from build123d import *

# Parameters (mm, degrees)
SKETCH1_W            = 15.8
SKETCH1_H            = 3.2
BOSS_EXTRUDE1_DEPTH  = 7.8
SKETCH2_R            = 2.4
BOSS_EXTRUDE2_DEPTH  = 1.6
LPATTERN1_COUNT      = 2
LPATTERN1_PITCH      = 8
LPATTERN1_COUNT_DIR2 = 6
LPATTERN1_PITCH_DIR2 = 8
SHELL1_T             = -1.2
SKETCH3_R            = 1.5
SKETCH3_R_2          = 0.6
BOSS_EXTRUDE3_DEPTH  = 1.8
BOSS_EXTRUDE4_DEPTH  = 1.5
SKETCH5_R            = 2.4
SKETCH5_R_2          = 1.55
BOSS_EXTRUDE5_DEPTH  = 1.6
LPATTERN2_COUNT      = 4
LPATTERN2_PITCH      = 8


with BuildPart() as part:
    # Sketch1 → Boss-Extrude1 (new body)
    with BuildSketch(Plane.XY):
        with Locations((7.9, 1.6)):
            Rectangle(SKETCH1_W, SKETCH1_H)
    extrude(amount=-BOSS_EXTRUDE1_DEPTH)

    # Sketch2 → Boss-Extrude2 (add)
    with BuildSketch(Plane(origin=(0, 3.2, 0), x_dir=(1, 0, 0), z_dir=(0, 1, 0))):
        with Locations(Location((3.9, 3.9, 0), (0, 0, 270))):
            Circle(SKETCH2_R)
    boss_extrude2 = extrude(amount=BOSS_EXTRUDE2_DEPTH)

    # LPattern1: Boss-Extrude2 2 × 6, 10 skipped
    with Locations(*[(j * LPATTERN1_PITCH_DIR2, 0, i * LPATTERN1_PITCH) for i in range(LPATTERN1_COUNT) for j in range(LPATTERN1_COUNT_DIR2) if (i, j) not in ((0, 0), (0, 2), (0, 3), (0, 4), (0, 5), (1, 0), (1, 1), (1, 2), (1, 3), (1, 4), (1, 5))]):
        add(boss_extrude2)

    # Shell1
    shell1_openings = [part.faces().sort_by_distance(p)[0] for p in [
        (7.9, 0, -3.9),
    ]]
    offset(amount=SHELL1_T, openings=shell1_openings, kind=Kind.INTERSECTION)

    # Sketch3 → Boss-Extrude3 (add)
    with BuildSketch(Plane.XZ.offset(-2)):
        with Locations(Location((7.9, -3.9, 0), (0, 0, 90))):
            Circle(SKETCH3_R)
        with Locations(Location((7.9, -3.9, 0), (0, 0, 270))):
            Circle(SKETCH3_R_2, mode=Mode.SUBTRACT)
    extrude(amount=BOSS_EXTRUDE3_DEPTH)

    # Sketch4 → Boss-Extrude4 (add)
    with BuildSketch(Plane(origin=(0, 0, -7.8), x_dir=(-1, 0, 0), z_dir=(0, 0, -1))):
        Polygon((-15.8, 3.2), (-23.8, 3.2), (-23.8, -4.6), (8, -4.6), (8, 3.2), (0, 3.2), align=None)
    extrude(amount=BOSS_EXTRUDE4_DEPTH)

    # Sketch5 → Boss-Extrude5 (add)
    with BuildSketch(Plane(origin=(0, 0, -9.3), x_dir=(-1, 0, 0), z_dir=(0, 0, -1))):
        with Locations((4.1, -0.7)):
            Circle(SKETCH5_R)
        with Locations((4.1, -0.7)):
            Circle(SKETCH5_R_2, mode=Mode.SUBTRACT)
    boss_extrude5 = extrude(amount=BOSS_EXTRUDE5_DEPTH)

    # LPattern2: Boss-Extrude5 ×4
    with Locations(*[(i * LPATTERN2_PITCH, 0, 0) for i in range(1, LPATTERN2_COUNT)]):
        add(boss_extrude5)


solid = part.part
Could you check a few things on this model? Use its own coordinates, in mm. A direction names the side the tool comes from. Round coordinates to 2 decimals unless told otherwise and drop trailing zeros. Write each loop counter-clockwise with the first axis right and the second up, starting at its lowest first coordinate (ties: lowest second). Pieces come first, ordered by that corner, then holes. Notation, with made-up numbers: (13, -27) - (40, -27) arc R31 cw to (40, 2) - close; hole circle Ø5 at (64, -11.75). An arc over 180 degrees is marked (long way). Put each result on its own line as item: value. Start each with the question number.
(1) For faces 1 (the flat face through (0, 2, -4)), 2 (the cylindrical face through (1.683, -1.619, -10.089)), 3 (the cylindrical face through (8.08, 1.113, -4.472)), which set-ups out of +Z, -Z, +X, -X, +Y, -Y let a thin tool reach every point of the face, with its end or its side?
(2) Will these pins go through, and if not, where does the flat tip stop? pin 1 (2.5 mm diameter, centred on x = 10.5, z = -3.5, fed in from -Y); pin 2 (0.6 mm diameter, centred on y = 1, z = -5, fed in from -X); pin 3 (2.5 mm diameter, centred on x = 12, z = -4, fed in from -Y).
(3) I want a section at B-B, the plane x = 7.9. Please give me the cut outline in (y, z).
(4) I want a section at D-D, the plane x = 11.9. Please give me the cut outline in (y, z).
(5) I need wall thicknesses on probe 1 along X at (y, z) = (2.45, -3.9); probe 2 along Z at (x, y) = (11.9, 3.1); probe 3 along Y at (x, z) = (-4.1, -10.5). Which ranges of each line are inside material? Lowest first, please.
(6) I want a section at A-A, the plane y = 2.5. Please give me the cut outline in (x, z).
(7) Thinking about a two-plate mould opening in Y: for faces 4 (the flat face through (-4, -1, -9.3)), 5 (the flat face through (8, 2, -4)), 6 (the cylindrical face through (10.422, -0.234, -10.089)), 7 (the cylindrical face through (13.09, 2.79, -4.06)), which applies, released by +Y, released by -Y, zero draft, split by the parting line, or undercut?
Here are the results:
1. face 1: +Z, -X, +Y, -Y
1. face 2: -Z
1. face 3: -Y
2. pin 1: stops at y = 0.2
2. pin 2: stops at x = 0
2. pin 3: stops at y = 2
3. outline: (-4.6, -9.3) - (3.2, -9.3) - (3.2, 0) - (0, 0) - (0, -1.2) - (2, -1.2) - (2, -2.4) - (0.2, -2.4) - (0.2, -3.3) - (2, -3.3) - (2, -4.5) - (0.2, -4.5) - (0.2, -5.4) - (2, -5.4) - (2, -6.6) - (0, -6.6) - (0, -7.8) - (-4.6, -7.8) - close
4. outline: (-4.6, -9.3) - (-3.1, -9.3) - (-3.1, -10.9) - (-2.25, -10.9) - (-2.25, -9.3) - (0.85, -9.3) - (0.85, -10.9) - (1.7, -10.9) - (1.7, -9.3) - (3.2, -9.3) - (3.2, -6.3) - (4.8, -6.3) - (4.8, -1.5) - (3.2, -1.5) - (3.2, 0) - (0, 0) - (0, -1.2) - (2, -1.2) - (2, -2.7) - (3.6, -2.7) - (3.6, -5.1) - (2, -5.1) - (2, -6.6) - (0, -6.6) - (0, -7.8) - (-4.6, -7.8) - close
5. probe 1: x = 0 to 2.7, 5.1 to 10.7, 13.1 to 15.8
5. probe 2: z = -9.3 to -5.1, -2.7 to 0
5. probe 3: y = -3.1 to -2.25, 0.85 to 1.7
6. outline: (-8, -9.3) - (23.8, -9.3) - (23.8, -7.8) - (15.8, -7.8) - (15.8, 0) - (0, 0) - (0, -7.8) - (-8, -7.8) - close; hole circle Ø2.4 at (3.9, -3.9); hole circle Ø2.4 at (11.9, -3.9)
7. face 4: undercut
7. face 5: released by -Y
7. face 6: undercut
7. face 7: zero draft
